The model under review builds one solid part; all positions refer to its coordinate system, in mm. A direction names the side the tool comes from. Give positions to 0.01 mm unless a question says otherwise; leave off trailing zeros. Loops run counter-clockwise (first coordinate to the right, second up) from the corner with the lowest first, then second, coordinate; pieces in that order, holes last. Notation, with made-up numbers: (18.5, 80.5) -> (70.5, 80.5) arc R12 ccw to (70.5, 103.5) -> close; hole circle Ø2 at (48.5, 63.25). An arc over 180 degrees is marked (long way). Write each question's results on one line, items separated by ' | '. Start each with the question number.
Q1. Machinability: for faces 4 (the face through (25, 21, 2)), 5 (the face through (20.943, 0.582, 1.972)), 6 (the face through (5, 42, 2)), 7 (the face through (14, 39, 2)), 8 (the face through (10, 36.75, 2)), which of the approach directions +Z, -Z, +X, -X, +Y, -Y give a long, thin tool a straight path to every point of the face, cutting with its end or side? Answer none if there is none.
Q2. Insertion check: pin 1 Ø1 at (x, z) = (14.5, 1) entering from -Y; pin 2 Ø2.5 at (x, y) = (4, 5) entering from -Z; pin 3 Ø1 at (x, z) = (21.5, 1) entering from -Y. Each pin has a flat end and moves straight along its axis. Give the tip position at first contact, or say it passes through.
Q3. We need section C-C (z = 3.2). Write out the cut boundary in (x, y).
Q4. Mouldability with a two-part tool opening along X and no side actions: class faces 1 (the face through (0, 21, 2)), 2 (the face through (24, 0, 2)), 3 (the face through (11, 32, 2)) as released by +X, released by -X, zero draft, split by the parting line, or undercut.
Q5. We need section A-A (y = 39.5). Write out the cut boundary in (x, z), plus the area to 3 significant figures.
Q6. We need section B-B (x = 14.5). Write out the cut boundary in (y, z), plus the area to 3 significant figures.
Q7. We need section D-D (y = 5). Write out the cut boundary in (x, z), plus the area to 3 significant figures.
Q8. Wall thickness on L1, parallel to Y at x = 21, z = 2.8; L2, parallel to Y at x = 4.25, z = 2.4; L3, parallel to X at y = 6, z = 0.5: over which ranges is each line inside the solid? List them lowest first. Write a range as [from, to].
from build123d import *

# Parameters (mm, degrees)
SKETCH_1_R      = 1.5
EXTRUDE_1_DEPTH = 4


with BuildPart() as part:
    # Эскиз1 → Бобышка-Вытянуть1 (new body)
    with BuildSketch(Plane.XY):
        with BuildLine():
            Line((11, 42), (11, 36.75))
            Line((11, 36.75), (9.75, 36.75))
            Line((9.75, 36.75), (9.75, 34.25))
            Line((9.75, 34.25), (11, 34.25))
            Line((11, 34.25), (11, 29))
            Line((11, 29), (14, 29))
            Line((14, 29), (14, 34.25))
            Line((14, 34.25), (15.25, 34.25))
            Line((15.25, 34.25), (15.25, 36.75))
            Line((15.25, 36.75), (14, 36.75))
            Line((14, 36.75), (14, 42))
            Line((14, 42), (25, 42))
            Line((25, 42), (25, 0))
            Line((25, 0), (22.718732798, 0))
            ThreePointArc((22.718732798, 0), (20.920846715, 0.598416016), (19.840216517, 2.154929577))
            ThreePointArc((19.840216517, 2.154929577), (12.5, 7.65), (5.159783483, 2.154929577))
            ThreePointArc((5.159783483, 2.154929577), (4.079153285, 0.598416016), (2.281267202, 0))
            Line((2.281267202, 0), (0, 0))
            Line((0, 0), (0, 42))
            Line((0, 42), (11, 42))
        make_face()
        with Locations((4, 5)):
            Circle(SKETCH_1_R, mode=Mode.SUBTRACT)
        with Locations((21, 5)):
            Circle(SKETCH_1_R, mode=Mode.SUBTRACT)
    extrude(amount=EXTRUDE_1_DEPTH)


solid = part.part
Output:
1) face 4: +Z, -Z, +X, +Y, -Y | face 5: +Z, -Z, -Y | face 6: +Z, -Z, +X, -X, +Y | face 7: +Z, -Z, +Y | face 8: +Z, -Z
2) pin 1: y = 7.23 | pin 2: through | pin 3: y = 0.09
3) outline: (0, 0) -> (2.28, 0) arc R3 ccw to (5.16, 2.15) arc R7.65 cw to (19.84, 2.15) arc R3 ccw to (22.72, 0) -> (25, 0) -> (25, 42) -> (14, 42) -> (14, 36.75) -> (15.25, 36.75) -> (15.25, 34.25) -> (14, 34.25) -> (14, 29) -> (11, 29) -> (11, 34.25) -> (9.75, 34.25) -> (9.75, 36.75) -> (11, 36.75) -> (11, 42) -> (0, 42) -> close; hole circle Ø3 at (4, 5); hole circle Ø3 at (21, 5)
4) face 1: released by -X | face 2: zero draft | face 3: undercut
5) outline: (0, 0) -> (11, 0) -> (11, 4) -> (0, 4) -> close; (14, 0) -> (25, 0) -> (25, 4) -> (14, 4) -> close | area: 88.0 mm2
6) outline: (7.38, 0) -> (34.25, 0) -> (34.25, 4) -> (7.38, 4) -> close; (36.75, 0) -> (42, 0) -> (42, 4) -> (36.75, 4) -> close | area: 128 mm2
7) outline: (0, 0) -> (2.5, 0) -> (2.5, 4) -> (0, 4) -> close; (5.5, 0) -> (6.71, 0) -> (6.71, 4) -> (5.5, 4) -> close; (18.29, 0) -> (19.5, 0) -> (19.5, 4) -> (18.29, 4) -> close; (22.5, 0) -> (25, 0) -> (25, 4) -> (22.5, 4) -> close | area: 29.7 mm2
8) L1: [0.54, 3.5], [6.5, 42] | L2: [0.74, 3.52], [6.48, 42] | L3: [0, 2.88], [5.12, 7.75], [17.25, 19.88], [22.12, 25]
